from build123d import *

# Parameters (mm, degrees)
SKETCH1_R           = 1.6
BOSS_EXTRUDE1_DEPTH = 8
SKETCH2_W           = 9
SKETCH2_H           = 8.199711987
CUT_EXTRUDE1_DEPTH  = 8
BOSS_EXTRUDE2_DEPTH = 6
SKETCH4_R           = 1.6
BOSS_EXTRUDE3_DEPTH = 8


with BuildPart() as part:
    # Sketch1 → Boss-Extrude1 (new body)
    with BuildSketch(Plane.XY):
        with BuildLine():
            Line((-0.5, 3), (15.5, 3))
            ThreePointArc((15.5, 3), (17.267766953, 2.267766953), (18, 0.5))
            Line((18, 0.5), (18, -0.5))
            ThreePointArc((18, -0.5), (17.267766953, -2.267766953), (15.5, -3))
            Line((15.5, -3), (-0.5, -3))
            ThreePointArc((-0.5, -3), (-2.267766953, -2.267766953), (-3, -0.5))
            Line((-3, -0.5), (-3, 0.5))
            ThreePointArc((-3, 0.5), (-2.267766953, 2.267766953), (-0.5, 3))
        make_face()
        Circle(SKETCH1_R, mode=Mode.SUBTRACT)
        with Locations((15, 0)):
            Circle(SKETCH1_R, mode=Mode.SUBTRACT)
    extrude(amount=BOSS_EXTRUDE1_DEPTH)

    # Sketch2 → Cut-Extrude1 (cut)
    with BuildSketch(Plane.XZ.offset(3)):
        with Locations((7.5, 6.099855994)):
            Rectangle(SKETCH2_W, SKETCH2_H)
    extrude(amount=-CUT_EXTRUDE1_DEPTH, mode=Mode.SUBTRACT)

    # Sketch3 → Boss-Extrude2 (add)
    with BuildSketch(Plane.XZ.offset(3)):
        Polygon((3.257359313, 2), (7.5, 6.242640687), (11.742640687, 2), align=None)
    extrude(amount=-BOSS_EXTRUDE2_DEPTH)

    # Sketch4 → Boss-Extrude3 (add)
    with BuildSketch(Plane(origin=(0, 0, 0), x_dir=(-1, 0, 0), z_dir=(0, 0, -1))):
        with BuildLine():
            ThreePointArc((8, 3), (9.767766953, 2.267766953), (10.5, 0.5))
            Line((10.5, 0.5), (10.5, -0.5))
            ThreePointArc((10.5, -0.5), (9.767766953, -2.267766953), (8, -3))
            Line((8, -3), (0.5, -3))
            ThreePointArc((0.5, -3), (2.267766953, -2.267766953), (3, -0.5))
            Line((3, -0.5), (3, 0.5))
            ThreePointArc((3, 0.5), (2.267766953, 2.267766953), (0.5, 3))
            Line((0.5, 3), (8, 3))
        make_face()
        with Locations((7.5, 0)):
            Circle(SKETCH4_R, mode=Mode.SUBTRACT)
        with BuildLine():
            ThreePointArc((-23, -3), (-24.767766953, -2.267766953), (-25.5, -0.5))
            Line((-25.5, -0.5), (-25.5, 0.5))
            ThreePointArc((-25.5, 0.5), (-24.767766953, 2.267766953), (-23, 3))
            Line((-23, 3), (-15.5, 3))
            ThreePointArc((-15.5, 3), (-17.267766953, 2.267766953), (-18, 0.5))
            Line((-18, 0.5), (-18, -0.5))
            ThreePointArc((-18, -0.5), (-17.267766953, -2.267766953), (-15.5, -3))
            Line((-15.5, -3), (-23, -3))
        make_face()
        with Locations((-22.5, 0)):
            Circle(SKETCH4_R, mode=Mode.SUBTRACT)
    extrude(amount=-BOSS_EXTRUDE3_DEPTH)


solid = part.part
Part model, mm, in its own coordinate system. A direction names the side the tool comes from. Give positions to 0.01 mm unless a question says otherwise; leave off trailing zeros. Write each loop counter-clockwise with the first axis right and the second up, starting at its lowest first coordinate (ties: lowest second). Pieces come first, ordered by that corner, then holes.
1) Probe L1, parallel to Y at x = -7.5, z = 5.5; L2, parallel to X at y = 2.75, z = 5; L3, parallel to X at y = 0.75, z = 1. List the from-to ranges inside material, lowest first.
Resolved:
L1: y = -3 to -1.6, 1.6 to 3
L2: x = -9.09 to 3, 6.26 to 8.74, 12 to 24.09
L3: x = -10.49 to -8.91, -6.09 to -1.41, 1.41 to 13.59, 16.41 to 21.09, 23.91 to 25.49
2) Cut at C-C on x = -7.5. Write the cut outline in (y, z).
Resolved:
outline: (-3, 0) - (-1.6, 0) - (-1.6, 8) - (-3, 8) - close; (1.6, 0) - (3, 0) - (3, 8) - (1.6, 8) - close
3) Cut at A-A on z = 6.75. Write the cut outline in (x, y).
Resolved:
outline: (-10.5, -0.5) arc R2.5 ccw to (-8, -3) - (3, -3) - (3, 3) - (-8, 3) arc R2.5 ccw to (-10.5, 0.5) - close; (12, -3) - (23, -3) arc R2.5 ccw to (25.5, -0.5) - (25.5, 0.5) arc R2.5 ccw to (23, 3) - (12, 3) - close; hole circle Ø3.2 at (-7.5, 0); hole circle Ø3.2 at (0, 0); hole circle Ø3.2 at (15, 0); hole circle Ø3.2 at (22.5, 0)
4) Cut at D-D on z = 5. Write the cut outline in (x, y).
Resolved:
outline: (-10.5, -0.5) arc R2.5 ccw to (-8, -3) - (3, -3) - (3, 3) - (-8, 3) arc R2.5 ccw to (-10.5, 0.5) - close; (6.26, -3) - (8.74, -3) - (8.74, 3) - (6.26, 3) - close; (12, -3) - (23, -3) arc R2.5 ccw to (25.5, -0.5) - (25.5, 0.5) arc R2.5 ccw to (23, 3) - (12, 3) - close; hole circle Ø3.2 at (-7.5, 0); hole circle Ø3.2 at (0, 0); hole circle Ø3.2 at (15, 0); hole circle Ø3.2 at (22.5, 0)
5) Cut at B-B on y = 0. Write the cut outline in (x, z).
Resolved:
outline: (-10.5, 0) - (-9.1, 0) - (-9.1, 8) - (-10.5, 8) - close; (-5.9, 0) - (-1.6, 0) - (-1.6, 8) - (-5.9, 8) - close; (1.6, 0) - (13.4, 0) - (13.4, 8) - (12, 8) - (12, 2) - (11.74, 2) - (7.5, 6.24) - (3.26, 2) - (3, 2) - (3, 8) - (1.6, 8) - close; (16.6, 0) - (20.9, 0) - (20.9, 8) - (16.6, 8) - close; (24.1, 0) - (25.5, 0) - (25.5, 8) - (24.1, 8) - close
6) Two-plate mould, pull along X, no slides. Class faces 3 (the face through (25, 2, 4)), 4 (the face through (-1.27, -0.97, 3.94)), 5 (the face through (19, 0, 8)): released by +X, released by -X, zero draft, split by the parting line, or undercut.
Resolved:
face 3: released by +X
face 4: undercut
face 5: zero draft
7) Which spindle directions (+Z, -Z, +X, -X, +Y, -Y) get a long thin tool onto all of the face, cutting with end or side? Do faces 1 (the face through (-10.5, 0, 4)), 2 (the face through (9.59, -0.04, 4.15)). Say none if no direction does.
Resolved:
face 1: +Z, -Z, -X, +Y, -Y
face 2: +Z, +Y, -Y
